Answer from the drawing. Dimensions are ordinates in mm from the lowest x, y and z of the part. A direction names the side the tool comes from. Give positions to 0.01 mm unless a question says otherwise; leave off trailing zeros. Write each loop counter-clockwise with the first axis right and the second up, starting at its lowest first coordinate (ties: lowest second). Pieces come first, ordered by that corner, then holes.
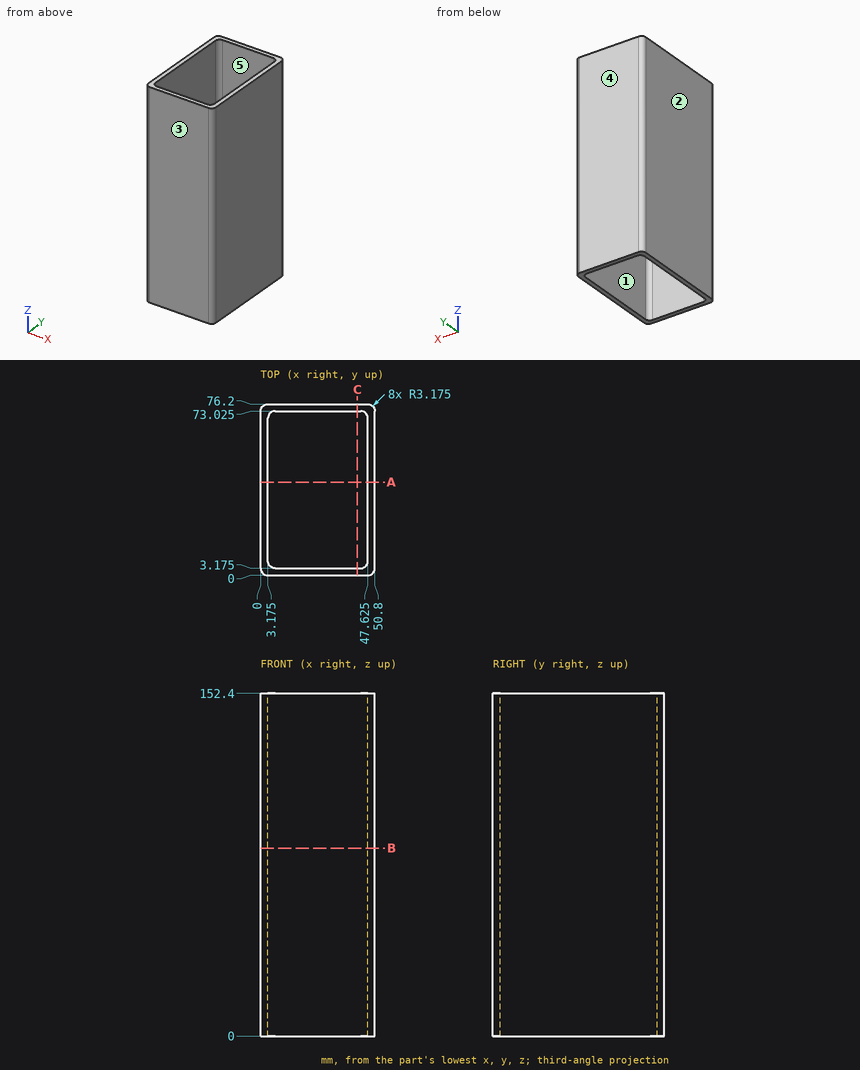
Item 1: Section A-A (y = 41.5) is taken. Write down the section's boundary in (x, z) (3 decimals).
Result set:
outline: (0, 0) - (3.175, 0) - (3.175, 152.4) - (0, 152.4) - close; (47.625, 0) - (50.8, 0) - (50.8, 152.4) - (47.625, 152.4) - close
Item 2: Find the intervals of material crossed by line 1 along X through (y, z) = (7.5, 56.5) (3 decimals); line 2 along Y through (x, z) = (34, 31) (3 decimals); line 3 along Y through (x, z) = (48, 28), in increasing order.
Result set:
line 1: x = 0 to 3.175, 47.625 to 50.8
line 2: y = 0 to 3.175, 73.025 to 76.2
line 3: y = 0.02 to 76.18
Item 3: Section C-C (x = 43) is taken. Write down the section's boundary in (y, z) (3 decimals), and give its area (3 significant figures).
Result set:
outline: (0, 0) - (3.175, 0) - (3.175, 152.4) - (0, 152.4) - close; (73.025, 0) - (76.2, 0) - (76.2, 152.4) - (73.025, 152.4) - close
area: 968 mm2
Item 4: Section B-B (z = 83.5) is taken. Write down the section's boundary in (x, y) (3 decimals), and give its area (3 significant figures).
Result set:
outline: (0, 3.175) arc R3.175 ccw to (3.175, 0) - (47.625, 0) arc R3.175 ccw to (50.8, 3.175) - (50.8, 73.025) arc R3.175 ccw to (47.625, 76.2) - (3.175, 76.2) arc R3.175 ccw to (0, 73.025) - close; hole (3.175, 6.35) arc R3.175 ccw to (6.35, 3.175) - (44.45, 3.175) arc R3.175 ccw to (47.625, 6.35) - (47.625, 69.85) arc R3.175 ccw to (44.45, 73.025) - (6.35, 73.025) arc R3.175 ccw to (3.175, 69.85) - close
area: 766 mm2
Item 5: Which of the six approach directions +Z, -Z, +X, -X, +Y, -Y give full straight-line access (tool end or side, diameter ignored) to the marked faces 1 and 2?
Result set:
face 1: +Z, -Z
face 2: +Z, -Z, -X, +Y, -Y
Item 6: Determine the mould class of the marked faces 3, 4 and 5 for opening direction Y: pulls with the +Y half, pulls with the -Y half, needs draft (parallel to the pull), parting line crosses it, or undercut.
Result set:
face 3: pulls with the -Y half
face 4: pulls with the +Y half
face 5: undercut
